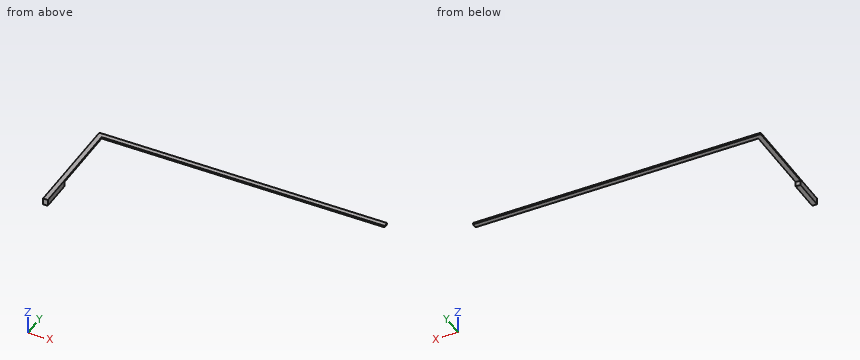
```python
from build123d import *

# Parameters (mm, degrees)
BOSS_EXTRUDE1_DEPTH = 5
SKETCH3_W           = 15
SKETCH3_H           = 100
BOSS_EXTRUDE2_DEPTH = 15


with BuildPart() as part:
    # Sketch1 → Boss-Extrude1 (new body)
    with BuildSketch(Plane.XY):
        Polygon((0, 0), (0, -340), (15, -340), (15, -14.996834209), (900, -14.996834209), (900, 0), align=None)
    extrude(amount=BOSS_EXTRUDE1_DEPTH)

    # Sketch3 → Boss-Extrude2 (add)
    with BuildSketch(Plane.XY):
        with Locations((7.5, -290)):
            Rectangle(SKETCH3_W, SKETCH3_H)
    extrude(amount=-BOSS_EXTRUDE2_DEPTH)


solid = part.part
```
The listing builds one solid part. Answer for the finished solid, in the listing's coordinates (mm). Give positions to 0.01 mm unless a question says otherwise; leave off trailing zeros. Write each loop counter-clockwise with the first axis right and the second up, starting at its lowest first coordinate (ties: lowest second). Pieces come first, ordered by that corner, then holes. Notation, with made-up numbers: M 87.25,24 L 100.25,24 A36 ccw 100.25,60 Z; hole C -14,23.25 d2. An arc over 180 degrees is marked long. Write each question's results on one line, items separated by ' | '.
Q1. Section B-B, the plane z = -3 is taken. Write down the section's boundary in (x, y).
Output values:
outline: M 0,-340 L 15,-340 L 15,-240 L 0,-240 Z
Q2. Flat-ended cylindrical pins translate along their axes: P1, Ø10, axis at y = -111, z = -1.5, coming from the +X side; P2, Ø7.5, axis at x = 7.5, z = -7, coming from the +Y side; P3, Ø4, axis at x = 637.5, z = 3.5, coming from the -Y side; P4, Ø2, axis at y = -200, z = -2, coming from the -X side. Find the tip coordinate at first contact, or state that the pin passes through.
Output values:
P1: x = 15 | P2: y = -240 | P3: y = -15 | P4: through
Q3. Section A-A, the plane y = -279.5 is taken. Write down the section's boundary in (x, z), then the cut area to 3 significant figures.
Output values:
outline: M 0,-15 L 15,-15 L 15,5 L 0,5 Z | area: 300 mm2
Q4. Consider L1, parallel to Y at x = 49.5, z = 2; L2, parallel to X at y = -151, z = 0.75. Determine where each line is inside the solid, lowest interval first. Write a range as from..to.
Output values:
L1: -15..0 | L2: 0..15
